Read the model definition and answer for the solid it produces. Units are mm, in the model's axes. A direction names the side the tool comes from. Round coordinates to 2 decimals unless told otherwise and drop trailing zeros. Order: outer loops, then holes, each group sorted by start corner. A loop starts at its lowest first (then second) coordinate and runs counter-clockwise, first axis right, second up. Notation, with made-up numbers: (37.25, 68) - (87.25, 68) arc R30 cw to (87.25, 94) - close; hole circle Ø11 at (60.25, 43). An arc over 180 degrees is marked (long way). One line per question, with ' | ' between items. Start each with the question number.
1) The part is cut by section C-C, the plane x = -17. Give the vertices of the cut face in (y, z).
2) For faces 1 (the cylindrical face through (17.744, 1.318, -1.579)), 2 (the cylindrical face through (-15.45, 1.65, 40.28)), determine the directions among +Z, -Z, +X, -X, +Y, -Y from which every point of the face is accessible in a straight line to the end or side of a thin tool.
3) Straight lines are drawn through the part: line 1 (X direction, y = 3.95, z = -35); line 2 (Z direction, x = 12.7, y = 2.4); line 3 (X direction, y = 2.15, z = -35). For each, find the intervals that lie inside material, in ascending order. Write a range as from..to.
4) The part is cut by section A-A, the plane z = -35. Give the vertices of the cut face in (x, y).
5) The mould has two halves that part along X. Classify faces 3 (the flat face through (0, 0, -1)), 4 (the flat face through (-25, 2, 1)), 5 (the cylindrical face through (-15.45, 1.65, -29.72)): pulls with the +X half, pulls with the -X half, needs draft (parallel to the pull), parting line crosses it, or undercut.
6) Flat-ended cylindrical pins translate along their axes: pin 1 (5 mm diameter, centred on x = -10.04, z = -13.09, fed in from +Y); pin 2 (6 mm diameter, centred on x = -15, z = 33.5, fed in from -Y); pin 3 (4 mm diameter, centred on x = 16.36, z = -2.15, fed in from +Y). Find the tip coordinate at first contact, or state that the pin passes through.
7) The part is cut by section B-B, the plane y = 4.2. Give the vertices of the cut face in (x, z), plus the area to 3 significant figures.
from build123d import *

# Parameters (mm, degrees)
SKETCH1_W                                        = 50
SKETCH1_H                                        = 100
BOSS_EXTRUDE1_DEPTH                              = 5
SKETCH3_R                                        = 1.5
CUT_EXTRUDE2_DEPTH                               = 5
CHAMFER1_SIZE                                    = 2.4
CBORE_FOR_1_4_BUTTON_HEAD_CAP_SCREW2_D           = 6.7564
CBORE_FOR_1_4_BUTTON_HEAD_CAP_SCREW2_CBORE_D     = 11.90752
CBORE_FOR_1_4_BUTTON_HEAD_CAP_SCREW2_CBORE_DEPTH = 3.3528


with BuildPart() as part:
    # Sketch1 → Boss-Extrude1 (new body)
    with BuildSketch(Plane(origin=(0, 0, 0), x_dir=(1, 0, 0), z_dir=(0, 1, 0))):
        Rectangle(SKETCH1_W, SKETCH1_H)
    extrude(amount=BOSS_EXTRUDE1_DEPTH)

    # Sketch3 → Cut-Extrude2 (cut)
    with BuildSketch(Plane(origin=(0, 5, 0), x_dir=(1, 0, 0), z_dir=(0, 1, 0))):
        with Locations((-6.314276634, -15.244012286)):
            Circle(SKETCH3_R)
        with Locations((16.358840213, 2.153682172)):
            Circle(SKETCH3_R)
        with Locations((-10.044563579, 13.090330115)):
            Circle(SKETCH3_R)
    extrude(amount=-CUT_EXTRUDE2_DEPTH, mode=Mode.SUBTRACT)

    # Chamfer1
    chamfer1_edges = [part.edges().sort_by_distance(p)[0] for p in [
        (-7.814276634, 5, 15.244012286),
        (14.858840213, 5, -2.153682172),
        (-11.544563579, 5, -13.090330115),
    ]]
    chamfer(chamfer1_edges, length=CHAMFER1_SIZE)

    # CBORE for 1/4 Button Head Cap Screw2 (through all)
    with Locations(Plane(origin=(0, 0, 0), x_dir=(-1, 0, 0), z_dir=(0, -1, 0))):
        with Locations((12.7, -35), (-12.7, -35), (-12.7, 35), (12.7, 35)):
            CounterBoreHole(CBORE_FOR_1_4_BUTTON_HEAD_CAP_SCREW2_D / 2, CBORE_FOR_1_4_BUTTON_HEAD_CAP_SCREW2_CBORE_D / 2, CBORE_FOR_1_4_BUTTON_HEAD_CAP_SCREW2_CBORE_DEPTH)


solid = part.part
Values:
1) outline: (0, -50) - (5, -50) - (5, 50) - (0, 50) - (0, 39.12) - (3.35, 39.12) - (3.35, 30.88) - (0, 30.88) - (0, -30.88) - (3.35, -30.88) - (3.35, -39.12) - (0, -39.12) - close
2) face 1: +Y, -Y | face 2: -Y
3) line 1: x = -25..-16.08, -9.32..9.32, 16.08..25 | line 2: z = -50..-40.95, -29.05..29.05, 40.95..50 | line 3: x = -25..-18.65, -6.75..6.75, 18.65..25
4) outline: (-25, 0) - (-18.65, 0) - (-18.65, 3.35) - (-16.08, 3.35) - (-16.08, 5) - (-25, 5) - close; (-9.32, 3.35) - (-6.75, 3.35) - (-6.75, 0) - (6.75, 0) - (6.75, 3.35) - (9.32, 3.35) - (9.32, 5) - (-9.32, 5) - close; (16.08, 3.35) - (18.65, 3.35) - (18.65, 0) - (25, 0) - (25, 5) - (16.08, 5) - close
5) face 3: needs draft | face 4: pulls with the -X half | face 5: undercut
6) pin 1: stops at y = 3.6 | pin 2: stops at y = 3.35 | pin 3: stops at y = 3.1
7) outline: (-25, -50) - (25, -50) - (25, 50) - (-25, 50) - close; hole circle Ø6.76 at (-12.7, -35); hole circle Ø6.76 at (-12.7, 35); hole circle Ø6.2 at (-10.04, -13.09); hole circle Ø6.2 at (-6.31, 15.24); hole circle Ø6.76 at (12.7, -35); hole circle Ø6.76 at (12.7, 35); hole circle Ø6.2 at (16.36, -2.15) | area: 4,770 mm^2
